Input: part model. Units: mm. Frame: model coordinates. Face numbers are marked on the shaded views. A direction names the side the tool comes from. Round coordinates to 2 decimals unless told otherwise and drop trailing zeros. Loops run counter-clockwise (first coordinate to the right, second up) from the corner with the lowest first, then second, coordinate; pieces in that order, holes last.
1) First-contact query: pin 1 (3.5 mm diameter, centred on x = 4, y = 1, fed in from +Z); pin 2 (3 mm diameter, centred on x = 5.5, z = 5, fed in from -Y); pin 3 (3 mm diameter, centred on x = -7.5, z = 4, fed in from -Y); pin 4 (6 mm diameter, centred on y = -3, z = -14, fed in from -X). Flat tips, straight axial feed; report the tip coordinate or a pass-through.
2) Draft query along Y for the marked faces 1, 2 and 3. Return one class per face: pulls with the +Y half, pulls with the -Y half, needs draft (parallel to the pull), parting line crosses it, or undercut.
3) Access query for the marked faces 4, 5 and 6. Directions: +Z, -Z, +X, -X, +Y, -Y. A direction counts if a zero-diameter tool reaches every point of the face in a straight line with its end or side. Return the directions, or none.
4) Ray query, line 1 along Z through (x, y) = (-7.1, 1); line 2 along Z through (x, y) = (-7.1, 0.5); line 3 along X through (y, z) = (-1.5, -16.25). Return the intervals inside material, ascending.
5) Section A-A, the plane x = 0.25. Return loops of the section in (y, z).
6) Section C-C, the plane y = -0.25. State how many separate pieces and enclosed holes the cut face has, and give its area (3 significant figures).
7) Section B-B, the plane x = -7.5. Return loops of the section in (y, z).
from build123d import *
from OCP.BRepFilletAPI import BRepFilletAPI_MakeChamfer

# Parameters (mm, degrees)
BOSS_EXTRUDE1_DEPTH             = 9.2
BOSS_EXTRUDE1_DEPTH_BACK        = 10
SKETCH1_W                       = 13.1
SKETCH1_H                       = 6.6
SKETCH2_W                       = 13.1
SKETCH2_H                       = 6.6
SKETCH2_R                       = 1.5
SKETCH2_W_2                     = 6.55
BOSS_EXTRUDE2_DEPTH             = 1.2
CUT_EXTRUDE1_DEPTH              = 20.4
FILLET1_R                       = 7
BOSS_EXTRUDE3_REACH             = 28.189
BOSS_EXTRUDE3_END_RADIUS        = 80
SKETCH4_R                       = 1.5
BOSS_EXTRUDE3_DIRECTION_2_DEPTH = 1
SKETCH5_R                       = 1.4
CUT_EXTRUDE2_DEPTH              = 7
CHAMFER1_SIZE                   = 0.25
CHAMFER1_SIZE2                  = 1.417820455
FILLET2_R                       = 0.5


with BuildPart() as part:
    # Sketch1 → Boss-Extrude1 (new, two sides: drawn at the far end of the back side and taken through both)
    with BuildSketch(Plane(origin=(0, 0, 0), x_dir=(0, 0, -1), z_dir=(1, 0, 0)).offset(-BOSS_EXTRUDE1_DEPTH_BACK)):
        Polygon((-8.75, -4), (-4.75, 8), (17.25, 8), (21.25, -4), align=None)
        with Locations((6.25, 2.5)):
            Rectangle(SKETCH1_W, SKETCH1_H, mode=Mode.SUBTRACT)
    extrude(amount=BOSS_EXTRUDE1_DEPTH + BOSS_EXTRUDE1_DEPTH_BACK)

    # Sketch2 → Boss-Extrude2 (add)
    # profile 1 of 3: a face of its own
    with BuildSketch(Plane(origin=(9.2, 0, 0), x_dir=(0, 0, -1), z_dir=(1, 0, 0))):
        Polygon((-4.75, 8), (-8.75, -4), (21.25, -4), (17.25, 8), align=None)
        with Locations((6.25, 2.5)):
            Rectangle(SKETCH2_W, SKETCH2_H, mode=Mode.SUBTRACT)
    # profile 2 of 3: a face of its own
    with BuildSketch(Plane(origin=(9.2, 0, 0), x_dir=(0, 0, -1), z_dir=(1, 0, 0))):
        with Locations((6.25, 2.5)):
            Rectangle(SKETCH2_W, SKETCH2_H)
        with Locations((2.975, 2.5)):
            Circle(SKETCH2_R, mode=Mode.SUBTRACT)
        with Locations((9.525, 2.5)):
            Circle(SKETCH2_R, mode=Mode.SUBTRACT)
    # profile 3 of 3: a face of its own
    with BuildSketch(Plane(origin=(9.2, 0, 0), x_dir=(0, 0, -1), z_dir=(1, 0, 0))):
        with Locations((9.525, 2.5)):
            Rectangle(SKETCH2_W_2, SKETCH2_H)
        with Locations((9.525, 2.5)):
            Circle(SKETCH2_R, mode=Mode.SUBTRACT)
    extrude(amount=BOSS_EXTRUDE2_DEPTH)

    # Sketch3 → Cut-Extrude1 (cut)
    with BuildSketch(Plane(origin=(10.4, 0, 0), x_dir=(0, 0, -1), z_dir=(1, 0, 0))):
        with BuildLine():
            Line((21.091886117, -3.525658351), (21.25, -4))
            Line((21.25, -4), (-8.75, -4))
            Line((-8.75, -4), (-8.591886117, -3.525658351))
            ThreePointArc((-8.591886117, -3.525658351), (6.25, -2.136843411), (21.091886117, -3.525658351))
        make_face()
    extrude(amount=-CUT_EXTRUDE1_DEPTH, mode=Mode.SUBTRACT)

    # Fillet1
    fillet1_edges = [part.edges().sort_by_distance(p)[0] for p in [
        (0.2, 8, 4.75),
        (0.2, 8, -17.25),
    ]]
    fillet(fillet1_edges, radius=FILLET1_R)

    # Boss-Extrude3: up to this cylinder (the profile starts inside it)
    boss_extrude3_end = Plane(origin=(3.4, -82.136843411, -6.25), z_dir=(1, 0, 0)) * Cylinder(BOSS_EXTRUDE3_END_RADIUS, 217.378, mode=Mode.PRIVATE)
    # Sketch4 → Boss-Extrude3 (add, up to the surface)
    with BuildSketch(Plane(origin=(0, -3.525658351, 0), x_dir=(1, 0, 0), z_dir=(0, 1, 0)), mode=Mode.PRIVATE) as boss_extrude3_sk1:
        with Locations(Location((3.4, 13.8, 0), (0, 0, 270))):
            Circle(SKETCH4_R)
    boss_extrude3_tool1 = extrude(boss_extrude3_sk1.sketch, amount=BOSS_EXTRUDE3_REACH, mode=Mode.PRIVATE) & boss_extrude3_end
    add(boss_extrude3_tool1.solids().sort_by_distance((3.4, -3.525658, -13.8))[0])
    # Sketch4 → Boss-Extrude3 (add, up to the surface)
    with BuildSketch(Plane(origin=(0, -3.525658351, 0), x_dir=(1, 0, 0), z_dir=(0, 1, 0)), mode=Mode.PRIVATE) as boss_extrude3_sk2:
        with Locations(Location((3.4, -1.3, 0), (0, 0, 270))):
            Circle(SKETCH4_R)
    boss_extrude3_tool2 = extrude(boss_extrude3_sk2.sketch, amount=BOSS_EXTRUDE3_REACH, mode=Mode.PRIVATE) & boss_extrude3_end
    add(boss_extrude3_tool2.solids().sort_by_distance((3.4, -3.525658, 1.3))[0])

    # Sketch4 → Boss-Extrude3 direction 2 (add)
    with BuildSketch(Plane(origin=(0, -3.525658351, 0), x_dir=(1, 0, 0), z_dir=(0, 1, 0))):
        with Locations(Location((3.4, 13.8, 0), (0, 0, 270))):
            Circle(SKETCH4_R)
        with Locations(Location((3.4, -1.3, 0), (0, 0, 270))):
            Circle(SKETCH4_R)
    extrude(amount=-BOSS_EXTRUDE3_DIRECTION_2_DEPTH)

    # Sketch5 → Cut-Extrude2 (cut)
    with BuildSketch(Plane(origin=(0, -3.525658351, 0), x_dir=(1, 0, 0), z_dir=(0, 1, 0))):
        with Locations(Location((-7.1, 16.25, 0), (0, 0, 90))):
            Circle(SKETCH5_R)
        with Locations(Location((-7.1, -3.75, 0), (0, 0, 90))):
            Circle(SKETCH5_R)
    extrude(amount=CUT_EXTRUDE2_DEPTH, mode=Mode.SUBTRACT)

    # Chamfer1: one chamfer whose edges measure the first distance from different faces: ONE call of the kernel's chamfer builder (chamfer() names one face for all edges)
    chamfer1_edges_1 = [part.edges().sort_by_distance(p)[0] for p in [
        (3.4, -4.525658351, -0.2),
    ]]
    chamfer1_side_1 = [part.faces().sort_by_distance(p)[0] for p in [
        (3.4, -4.525658351, 1.3),
    ]]
    chamfer1_edges_2 = [part.edges().sort_by_distance(p)[0] for p in [
        (3.4, -4.525658351, -15.3),
    ]]
    chamfer1_side_2 = [part.faces().sort_by_distance(p)[0] for p in [
        (3.4, -4.525658351, -13.8),
    ]]
    chamfer1 = BRepFilletAPI_MakeChamfer(part.part.solid().wrapped)
    for e in chamfer1_edges_1:
        chamfer1.Add(CHAMFER1_SIZE, CHAMFER1_SIZE2, e.wrapped, chamfer1_side_1[0].wrapped)  # the first distance lies on this face
    for e in chamfer1_edges_2:
        chamfer1.Add(CHAMFER1_SIZE, CHAMFER1_SIZE2, e.wrapped, chamfer1_side_2[0].wrapped)  # the first distance lies on this face
    add(Compound.cast(chamfer1.Shape()), mode=Mode.REPLACE)

    # Fillet2
    fillet2_edges = [part.edges().sort_by_distance(p)[0] for p in [
        (10.4, -0.156031994, -19.968677331),
        (-10, -0.156031994, -19.968677331),
        (10.4, -2.136843411, -6.25),
        (0.2, -3.525658351, -21.091886117),
        (0.2, -3.525658351, 8.591886117),
        (10.4, 8, -6.25),
        (10.4, -0.156031994, 7.468677331),
        (10.4, 6.678695296, 3.797657452),
        (10.4, 6.678695296, -16.297657452),
        (-10, 8, -6.25),
        (-10, -0.156031994, 7.468677331),
        (-10, 6.678695296, 3.797657452),
        (-10, 6.678695296, -16.297657452),
    ]]
    fillet(fillet2_edges, radius=FILLET2_R)


solid = part.part
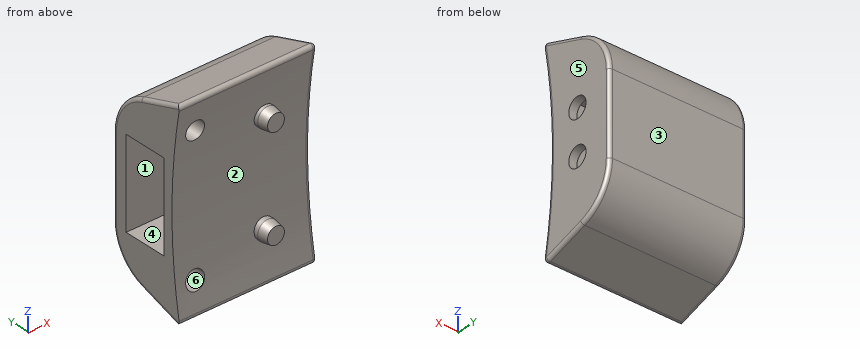
Final values:
1. pin 1: stops at z = 7.67
1. pin 2: stops at y = -3.16
1. pin 3: stops at y = -3
1. pin 4: stops at x = -10
2. face 1: undercut
2. face 2: pulls with the -Y half
2. face 3: pulls with the +Y half
3. face 4: -X
3. face 5: +Z, -Z, +X, +Y, -Y
3. face 6: -Y
4. line 1: z = -19.58 to -17.65, -14.85 to -12.8, 0.3 to 2.35, 5.15 to 7.08
4. line 2: z = -19.75 to -17.65, -14.85 to -12.8, 0.3 to 2.35, 5.15 to 7.25
4. line 3: x = -10 to -8.5, -5.7 to 10.4
5. outline: (-3.37, -20.26) arc R0.5 ccw to (-2.72, -20.82) - (3.21, -18.85) arc R7 ccw to (8, -12.2) - (8, -0.3) arc R7 ccw to (3.21, 6.35) - (-2.72, 8.32) arc R0.5 ccw to (-3.37, 7.76) arc R80 cw to start; hole (-0.8, -12.8) - (5.8, -12.8) - (5.8, 0.3) - (-0.8, 0.3) - close
6. separate pieces: 1
6. enclosed holes: 2
6. area: 297 mm2
7. outline: (-3.37, -20.26) arc R0.5 ccw to (-2.72, -20.82) - (3.21, -18.85) arc R7 ccw to (8, -12.2) - (8, -0.3) arc R7 ccw to (3.21, 6.35) - (-2.72, 8.32) arc R0.5 ccw to (-3.37, 7.76) arc R80 cw to (-2.94, 5.09) - (3.47, 5.09) - (3.47, 2.41) - (-2.61, 2.41) arc R80 cw to (-2.61, -14.91) - (3.47, -14.91) - (3.47, -17.59) - (-2.94, -17.59) arc R80 cw to start; hole (-0.8, -12.8) - (5.8, -12.8) - (5.8, 0.3) - (-0.8, 0.3) - close
